from build123d import *

# Parameters (mm, degrees)
BOX014_W                                          = 8
BOX014_H                                          = 10
BOX014_DEPTH                                      = 4.1
PRISM009_DEPTH                                    = 4.2
CYLINDER014005916_R                               = 3.65
CYLINDER014005916_DEPTH                           = 10
CYLINDER014005905_R                               = 2.65
CYLINDER014005905_DEPTH                           = 22.5
FUSION001089102007007003008034017_PLACEMENT_ANGLE = 120


with BuildPart() as krychle014:
    # Box014 → Box014 (new body)
    with BuildSketch(Plane(origin=(-3.5, 0, 7), x_dir=(1, 0, 0), z_dir=(0, 0, 1))):
        with Locations((4, 5)):
            Rectangle(BOX014_W, BOX014_H)
    extrude(amount=BOX014_DEPTH)


with BuildPart() as m4x005:
    # prism009 → prism009 (new body)
    with BuildSketch(Plane(origin=(0, 0, 7), x_dir=(0, 1, 0), z_dir=(0, 0, 1))):
        Polygon((4.6, 0), (2.3, 3.983717), (-2.3, 3.983717), (-4.6, 0), (-2.3, -3.983717), (2.3, -3.983717), align=None)
    extrude(amount=PRISM009_DEPTH)


with BuildPart() as obj1:
    # Cylinder014005916 → Cylinder014005916 (new body)
    with BuildSketch(Plane.XY.offset(-8)):
        Circle(CYLINDER014005916_R)
    extrude(amount=CYLINDER014005916_DEPTH)


with BuildPart() as m4nut014:
    # Cylinder014005905 → Cylinder014005905 (new body)
    with BuildSketch(Plane.XY.offset(-8)):
        Circle(CYLINDER014005905_R)
    extrude(amount=CYLINDER014005905_DEPTH)

    # Fusion001089102007007003008034015: union Krychle014, M4X005, obj1
    add(krychle014.part)
    add(m4x005.part)
    add(obj1.part)


with BuildPart() as m4nut014_1:
    # Fusion001089102007007003008034015 placement: moved
    add(m4nut014.part.moved(Location((0, -45, 0))))


with BuildPart() as m4nut014_2:
    # Fusion001089102007007003008034017 placement: moved
    add(m4nut014_1.part.rotate(Axis((0, 0, 0), (0, 0, 1)), FUSION001089102007007003008034017_PLACEMENT_ANGLE))


solid = m4nut014_2.part
Can you work these out from the model? Positions are in its coordinate system, mm. A direction names the side the tool comes from. Round coordinates to 2 decimals unless told otherwise and drop trailing zeros. Write each loop counter-clockwise with the first axis right and the second up, starting at its lowest first coordinate (ties: lowest second). Pieces come first, ordered by that corner, then holes. Notation, with made-up numbers: (39.25, -1.75) -> (88.25, -1.75) arc R16 ccw to (88.25, 6.25) -> close; hole circle Ø2 at (-32, -13.75). An arc over 180 degrees is marked (long way). Use one line per item in the form item = value. Start each with the question number.
Q1. Imagine slicing it at C-C (z = 8.5). Please give me the cut outline in (x, y).
Q2. If I drill on probe 1 along Z at (x, y) = (36.5, 25.25); probe 2 along Z at (x, y) = (34.25, 18.5); probe 3 along Y at (x, z) = (41.5, 7.5), over which ranges is the centre line in solid material (lowest first)? Write a range as [from, to].
Q3. Imagine slicing it at B-B (y = 21.75). Please give me the cut outline in (x, z), then the cut area to 3 significant figures.
Q4. We'd pull the mould along X, two halves only. Please class faces 1 (the face through (37.892, 26.477, 9.071)), 2 (the face through (35, 20, 7)), 3 (the face through (32.45, 23.93, 9.02)): +X half, -X half, draft (parallel to the pull), parting line (faces both ways), or undercut.
Q5. Imagine slicing it at D-D (x = 39.5). Please give me the cut outline in (y, z).
Q6. I'm going to push flat-ended pins straight in: P1, Ø1.5, axis at y = 23.5, z = 9, coming from the -X side; P2, Ø1.5, axis at x = 41.5, z = 8.5, coming from the -Y side; P3, Ø3, axis at x = 31.5, y = 21, coming from the +Z side. Where does each tip first touch, or does it pass through?
Q7. Which directions (+Z, -Z, +X, -X, +Y, -Y) give clear straight access to the entire face, cutting with the end or side of a thin tool? Please do faces 4 (the face through (36, 23, 2)), 5 (the face through (39.5, 19.7, 11.2)), 6 (the face through (38.741, 18.033, 9.557)), 7 (the face through (35.325, 22.66, -3.07)).
Q8. Imagine slicing it at A-A (x = 42). Please give me the cut outline in (y, z).
Worked out:
q1.outline = (28.06, 21.4) -> (32.06, 14.47) -> (38.49, 18.18) -> (38.97, 17.9) -> (42.95, 20.2) -> (42.95, 24.8) -> (38.97, 27.1) -> (36.98, 25.95) -> (36.72, 26.4) -> close
q2.probe_1 = [7, 11.2]
q2.probe_2 = [7, 11.1]
q2.probe_3 = [19.36, 25.64]
q3.outline = (28.67, 7) -> (36.43, 7) -> (36.43, 2) -> (35.4, 2) -> (35.4, -8) -> (42.54, -8) -> (42.54, 2) -> (41.51, 2) -> (41.51, 7) -> (42.95, 7) -> (42.95, 11.2) -> (41.51, 11.2) -> (41.51, 14.5) -> (36.43, 14.5) -> (36.43, 11.2) -> (34.99, 11.2) -> (34.99, 11.1) -> (28.67, 11.1) -> close
q3.area = 173 mm^2
q4.face_1 = undercut
q4.face_2 = draft
q4.face_3 = -X half
q5.outline = (18.21, 7) -> (19.9, 7) -> (19.9, 2) -> (18.89, 2) -> (18.89, -8) -> (26.11, -8) -> (26.11, 2) -> (25.1, 2) -> (25.1, 7) -> (26.79, 7) -> (26.79, 11.2) -> (25.1, 11.2) -> (25.1, 14.5) -> (19.9, 14.5) -> (19.9, 11.2) -> (18.21, 11.2) -> close
q6.P1 = 30.4
q6.P2 = 18.93
q6.P3 = 11.1
q7.face_4 = none
q7.face_5 = +Z
q7.face_6 = +Z, -Y
q7.face_7 = -Z
q8.outline = (19.65, 7) -> (25.35, 7) -> (25.35, 11.2) -> (19.65, 11.2) -> close; (20.46, -8) -> (24.54, -8) -> (24.54, 2) -> (20.46, 2) -> close
